Could you check a few things on this model? Use its own coordinates, in mm. A direction names the side the tool comes from. Give positions to 0.01 mm unless a question says otherwise; leave off trailing zeros. Write each loop counter-clockwise with the first axis right and the second up, starting at its lowest first coordinate (ties: lowest second). Pieces come first, ordered by that corner, then holes. Notation, with made-up numbers: M 43.5,75 L 101.5,75 A18 ccw 101.5,102 Z; hole C 34.25,86.5 d7. An arc over 180 degrees is marked long. Answer as CSV lines item,"result". Start each with the question number.
Autodesk Inventor part; units mm, degrees
ref_plane "YZ Plane" through (0, 0, 0) normal (1, 0, 0) x (0, 1, 0)
ref_plane "XZ Plane" through (0, 0, 0) normal (0, 1, 0) x (-1, 0, 0)
ref_plane "XY Plane" through (0, 0, 0) normal (0, 0, 1) x (1, 0, 0)
sketch "Sketch1" plane through (0, 0, 0) normal (0, 0, 1) x (1, 0, 0)
  line L0 (0, 0) -> (121, 0)
  line L1 (121, 0) -> (121, 60)
  line L2 (121, 60) -> (0, 60)
  line L3 (0, 60) -> (0, 0)
  dimension "d0" = 121
  dimension "d1" = 60
extrude "Extrusion1" add sketch "Sketch1" along normal blind 5
sketch "Sketch2" plane through (0, 0, 5) normal (0, 0, 1) x (1, 0, 0)
  circle A0 centre (60.5, 45.5856) radius 9.2358
  line L0 (121, 60) -> (0, 60) construction
  line L1 (60.5, 60) -> (60.5, 0) construction
  line L2 (0, 0) -> (121, 0) construction
extrude "Extrusion2" cut sketch "Sketch2" against normal blind 5
sketch "Sketch4" plane through (0, 0, 5) normal (0, 0, 1) x (1, 0, 0)
  circle A0 centre (60.5, 31) radius 16 construction
  line L0 (0, 0) -> (121, 0) construction
  line L1 (60.5, 0) -> (60.5, 60) construction
  line L2 (60.5, 60) -> (34.5, 60) construction
  arc A1 (39.5, 31) -> (81.5, 31) centre (60.5, 31) ccw
  line L3 (60.5, 31) -> (81.5, 31) construction
  line L4 (60.5, 31) -> (39.5, 31) construction
  line L5 (60.5, 60) -> (86.5, 60) construction
  line L6 (121, 60) -> (0, 60) construction
  line L7 (34.5, 60) -> (86.5, 60)
  arc A2 (39.5, 31) -> (34.5, 60) centre (-47.1, 31) ccw
  arc A3 (86.5, 60) -> (81.5, 31) centre (168.1, 31) ccw
  dimension "d28" = 26
  dimension "d30" = 21
  dimension "d33" = 32
  dimension "d34" = 180
  dimension "d35" = 90
  dimension "d36" = 26
  dimension "d39" = 0
extrude "Extrusion5" cut sketch "Sketch4" against normal blind 5
equation "\"d0\" = tankw + 2 * slack + 2 * surroundt + 2 * pvct"
equation "\"d1\" = surroundh"
equation "\"d2\" = surroundt"
equation "\"d4\" = surroundt"
equation "\"d30\" = 0.5 * diasurroundhole"
equation "\"d37\" = surroundt"
equation "\"lcsd\" = 19.05"
equation "\"lcwd1\" = 25"
equation "\"lcwd2\" = 34"
equation "\"lch1\" = 39"
equation "\"lcwd3\" = 43"
equation "\"dia1\" = 6"
equation "\"td\" = 18"
equation "\"bhh\" = 6"
equation "\"sw\" = 25"
equation "\"sh\" = 31"
equation "\"spacert\" = 2"
equation "\"pvct\" = 5"
equation "\"tankl\" = 379"
equation "\"dia4\" = 11"
equation "\"dia3\" = 8"
equation "\"play\" = 9"
equation "\"holeh\" = 26"
equation "\"surroundh\" = 60"
equation "\"slack\" = 0.5"
equation "\"surroundt\" = 5"
equation "\"play2\" = 3"
equation "\"diaair\" = 32"
equation "\"diacucl\" = 32"
equation "\"diawater\" = 25"
equation "\"diaph\" = 32"
equation "\"diaoverflow\" = 25"
equation "\"diasurroundhole\" = 42"
equation "\"diagrate\" = 12"
equation "\"gratespacing\" = 12.02082"
equation "\"bottomdist\" = 9.6355"
equation "\"sidedist\" = 13.9375"
equation "\"diahcl\" = 32"
equation "\"bracketwtop\" = 6"
equation "\"bracketwbottom\" = 6"
equation "\"nett\" = 1"
equation "\"nethole\" = 16"
equation "\"nettop\" = 7"
equation "\"netside\" = 3.5"
equation "\"netholespacing\" = 2"
equation "\"diaetape\" = 32"
properties part number "surround_front back" material "PVC-Piping"
1. Please list where these lines run through material, in increasing order: line 1 (X direction, y = 30, z = 1.5); line 2 (X direction, y = 17, z = 1.15); line 3 (Y direction, x = 59, z = 1.1).
2. Imagine slicing it at A-A, the plane y = 22.5. Please give me the cut outline in (x, z), plus the area to 3 significant figures.
3. On a 3-axis mill with a long thin cutter (end or side, diameter ignored), from which of +Z, -Z, +X, -X, +Y, -Y can I reach the whole of each face in a straight line? I mean faces 4 (the flat face through (46, 10, 0)), 5 (the cylindrical face through (82.795, 45.918, 2.535)). Say none if no direction works.
4. Imagine slicing it at B-B, the plane z = 2. Please give me the cut outline in (x, y), plus the area to 3 significant figures.
5. Will this pin go through, and if not, where does the flat tip stop? P1, Ø1, axis at x = 47, z = 4, coming from the +Y side.
6. Imagine slicing it at C-C, the plane x = 60.5. Please give me the cut outline in (y, z), plus the area to 3 significant figures.
7. Imagine slicing it at D-D, the plane y = 52.5. Please give me the cut outline in (x, z).
8. Thinking about a two-plate mould opening in X: for faces 1 (the flat face through (104, 60, 2)), 2 (the flat face through (0, 30, 2)), 3 (the cylindrical face through (38.276, 45.51, 2.535)), which applies, pulls with the +X half, pulls with the -X half, needs draft (parallel to the pull), parting line crosses it, or undercut?
Solutions:
1,line 1,"0 to 39.52, 81.48 to 121"
1,line 2,"0 to 44.85, 76.15 to 121"
1,line 3,"0 to 10.05"
2,outline,"M 0,0 L 41.3,0 L 41.3,5 L 0,5 Z; M 79.7,0 L 121,0 L 121,5 L 79.7,5 Z"
2,area,"413 mm²"
3,face 4,"-Z, +X, -X, +Y, -Y"
3,face 5,"+Z, -Z, +Y"
4,outline,"M 0,0 L 121,0 L 121,60 L 86.5,60 A86.6 ccw 81.5,31 A21 cw 39.5,31 A86.6 ccw 34.5,60 L 0,60 Z"
4,area,"5,250 mm²"
5,P1,"y = 15.35"
6,outline,"M 0,0 L 10,0 L 10,5 L 0,5 Z"
6,area,"50.0 mm²"
7,outline,"M 0,0 L 36.79,0 L 36.79,5 L 0,5 Z; M 84.21,0 L 121,0 L 121,5 L 84.21,5 Z"
8,face 1,"needs draft"
8,face 2,"pulls with the -X half"
8,face 3,"undercut"
